```python
from build123d import *
from build123d.topology import SkipClean

# Parameters (mm, degrees)
SKETCH1_R             = 22.146000031
BOSS_EXTRUDE1_DEPTH   = 19.05
SKETCH1_R_2           = 32.595999959
BOSS_EXTRUDE1_2_DEPTH = 19.05
SKETCH1_W             = 304.8
SKETCH1_H             = 304.8
SKETCH1_R_3           = 27.229000025
SKETCH1_R_4           = 38.354
SKETCH1_R_5           = 1.651
BOSS_EXTRUDE1_3_DEPTH = 19.05
SKETCH1_4_R           = 27.229000025
SKETCH1_4_R_2         = 22.146000031
SKETCH1_4_R_3         = 38.354
SKETCH1_4_R_4         = 32.595999959
BOSS_EXTRUDE2_DEPTH   = 12.7
SKETCH1_5_R           = 1.651
CUT_EXTRUDE1_DEPTH    = 12.7
SKETCH5_R             = 2.032
SKETCH5_R_2           = 2.38125
CUT_EXTRUDE2_DEPTH    = 13.7


with BuildPart() as part:
    # Sketch1 → Boss-Extrude1 (new body)
    with BuildSketch(Plane(origin=(0, 0, 0), x_dir=(1, 0, 0), z_dir=(0, 1, 0))):
        with Locations(Location((-11.176, 42.164, 0), (0, 0, 270))):  # turned: the seam where the file's is
            Circle(SKETCH1_R)
    extrude(amount=BOSS_EXTRUDE1_DEPTH)



with BuildPart() as body_2:
    # Sketch1 → Boss-Extrude1 2 (new body)
    with BuildSketch(Plane(origin=(0, 0, 0), x_dir=(1, 0, 0), z_dir=(0, 1, 0))):
        with Locations(Location((61.214, -20.32, 0), (0, 0, 270))):  # turned: the seam where the file's is
            Circle(SKETCH1_R_2)
    extrude(amount=BOSS_EXTRUDE1_2_DEPTH)


with BuildPart() as body_3:
    # Sketch1 → Boss-Extrude1 3 (new body)
    with BuildSketch(Plane(origin=(0, 0, 0), x_dir=(1, 0, 0), z_dir=(0, 1, 0))):
        Rectangle(SKETCH1_W, SKETCH1_H)
        with Locations(Location((-11.176, 42.164, 0), (0, 0, 270))):  # turned: the seam where the file's is
            Circle(SKETCH1_R_3, mode=Mode.SUBTRACT)
        with Locations(Location((61.214, -20.32, 0), (0, 0, 270))):  # turned: the seam where the file's is
            Circle(SKETCH1_R_4, mode=Mode.SUBTRACT)
        with Locations(Location((0, 0, 0), (0, 0, 270))):  # turned: the seam where the file's is
            Circle(SKETCH1_R_5, mode=Mode.SUBTRACT)
    extrude(amount=BOSS_EXTRUDE1_3_DEPTH)


with BuildPart() as part_1:
    with SkipClean():  # keep this step's faces unmerged: merging them makes the solid invalid here
        add(part.part)

        add(body_2.part)  # Boss-Extrude2 merges body 2

        add(body_3.part)  # Boss-Extrude2 merges body 3
        # Sketch1_4 → Boss-Extrude2 (add)
        with BuildSketch(Plane(origin=(0, 0, 0), x_dir=(1, 0, 0), z_dir=(0, 1, 0))):
            with Locations(Location((-11.176, 42.164, 0), (0, 0, 270))):  # turned: the seam where the file's is
                Circle(SKETCH1_4_R)
            with Locations(Location((-11.176, 42.164, 0), (0, 0, 270))):  # turned: the seam where the file's is
                Circle(SKETCH1_4_R_2, mode=Mode.SUBTRACT)
            with Locations(Location((61.214, -20.32, 0), (0, 0, 270))):  # turned: the seam where the file's is
                Circle(SKETCH1_4_R_3)
            with Locations(Location((61.214, -20.32, 0), (0, 0, 270))):  # turned: the seam where the file's is
                Circle(SKETCH1_4_R_4, mode=Mode.SUBTRACT)
            with BuildLine():
                ThreePointArc((99.568, -20.32), (91.665349034, 2.998333088), (71.214, 16.707413034))
                Line((71.214, 16.707413034), (71.214, 10.704171437))
                ThreePointArc((71.214, 10.704171437), (87.562237255, -1.129648079), (93.809999959, -20.32))
                ThreePointArc((93.809999959, -20.32), (42.023648079, -46.668237255), (51.214, 10.704171437))
                Line((51.214, 10.704171437), (51.214, 16.707413034))
                ThreePointArc((51.214, 16.707413034), (37.895666912, -50.771349034), (99.568, -20.32))
            make_face()
            with BuildLine():
                Line((71.214, 10.704171437), (71.214, 16.707413034))
                ThreePointArc((71.214, 16.707413034), (61.214, 18.034), (51.214, 16.707413034))
                Line((51.214, 16.707413034), (51.214, 10.704171437))
                ThreePointArc((51.214, 10.704171437), (61.214, 12.275999959), (71.214, 10.704171437))
            make_face()
            with BuildLine():
                ThreePointArc((-1.176, 67.490240194), (-11.176, 69.393000025), (-21.176, 67.490240194))
                Line((-21.176, 67.490240194), (-21.176, 61.923689202))
                ThreePointArc((-21.176, 61.923689202), (-11.176, 64.310000031), (-1.176, 61.923689202))
                Line((-1.176, 61.923689202), (-1.176, 67.490240194))
            make_face()
            with BuildLine():
                Line((-21.176, 61.923689202), (-21.176, 67.490240194))
                ThreePointArc((-21.176, 67.490240194), (-26.491489579, 19.650576864), (16.053000025, 42.164))
                ThreePointArc((16.053000025, 42.164), (11.337423136, 57.479489579), (-1.176, 67.490240194))
                Line((-1.176, 67.490240194), (-1.176, 61.923689202))
                ThreePointArc((-1.176, 61.923689202), (7.690707684, 53.761096987), (10.970000031, 42.164))
                ThreePointArc((10.970000031, 42.164), (-22.773096987, 23.297292316), (-21.176, 61.923689202))
            make_face()
        extrude(amount=BOSS_EXTRUDE2_DEPTH)

    # Sketch1_5 → Cut-Extrude1 (cut)
    with SkipClean():  # keep this step's faces unmerged: merging them makes the solid invalid here
        with BuildSketch(Plane(origin=(0, 0, 0), x_dir=(1, 0, 0), z_dir=(0, 1, 0))):
            Polygon((-124.40847096, -109.680850921), (-152.4, -109.680850921), (-152.4, -152.4), (-109.680850921, -152.4), (-109.680850921, -124.40847096), align=None)
            with BuildLine():
                ThreePointArc((71.214, 16.707413034), (68.771077011, 30.302427293), (61.747960937, 42.196464709))
                Line((61.747960937, 42.196464709), (25.136544704, 84.689638699))
                ThreePointArc((25.136544704, 84.689638699), (-3.999588367, 92.191814566), (-21.176, 67.490240194))
                Line((-21.176, 67.490240194), (-21.176, 61.923689202))
                ThreePointArc((-21.176, 61.923689202), (-11.176, 64.310000031), (-1.176, 61.923689202))
                Line((-1.176, 61.923689202), (-1.176, 67.490240194))
                ThreePointArc((-1.176, 67.490240194), (2.963287054, 73.442991513), (9.984708116, 71.635066779))
                Line((9.984708116, 71.635066779), (31.14615486, 47.073956315))
                ThreePointArc((31.14615486, 47.073956315), (32.128503793, 44.270491708), (30.940983624, 41.547585342))
                Line((30.940983624, 41.547585342), (-27.66770876, -17.061107042))
                Line((-27.66770876, -17.061107042), (-118.661107042, -17.061107042))
                Line((-118.661107042, -17.061107042), (-118.661107042, -109.680850921))
                Line((-118.661107042, -109.680850921), (-109.680850921, -118.661107042))
                Line((-109.680850921, -118.661107042), (-17.061107042, -118.661107042))
                Line((-17.061107042, -118.661107042), (-17.061107042, -27.66770876))
                Line((-17.061107042, -27.66770876), (40.331599468, 29.72499775))
                ThreePointArc((40.331599468, 29.72499775), (43.35605702, 30.912517919), (46.284134621, 29.504004806))
                Line((46.284134621, 29.504004806), (46.596124349, 29.141892789))
                ThreePointArc((46.596124349, 29.141892789), (50.022253958, 23.339551873), (51.214, 16.707413034))
                Line((51.214, 16.707413034), (51.214, 10.704171437))
                ThreePointArc((51.214, 10.704171437), (61.214, 12.275999959), (71.214, 10.704171437))
                Line((71.214, 10.704171437), (71.214, 16.707413034))
            make_face()
            with Locations(Location((0, 0, 0), (0, 0, 270))):  # turned: the seam where the file's is
                Circle(SKETCH1_5_R, mode=Mode.SUBTRACT)
        extrude(amount=CUT_EXTRUDE1_DEPTH, mode=Mode.SUBTRACT)

    # Sketch5 → Cut-Extrude2 (cut, through all)
    with SkipClean():  # keep this step's faces unmerged: merging them makes the solid invalid here
        with BuildSketch(Plane(origin=(0, 12.7, 0), x_dir=(1, 0, 0), z_dir=(0, 1, 0))):
            with Locations(Location((-11.176, 17.476499972, 0), (0, 0, 270))):  # turned: the seam where the file's is
                Circle(SKETCH5_R)
            with Locations(Location((13.511500028, 42.164, 0), (0, 0, 270))):  # turned: the seam where the file's is
                Circle(SKETCH5_R)
            with Locations(Location((-35.863500028, 42.164, 0), (0, 0, 270))):  # turned: the seam where the file's is
                Circle(SKETCH5_R)
            with Locations(Location((25.739000021, -20.32, 0), (0, 0, 270))):  # turned: the seam where the file's is
                Circle(SKETCH5_R_2)
            with Locations(Location((96.68899998, -20.32, 0), (0, 0, 270))):  # turned: the seam where the file's is
                Circle(SKETCH5_R_2)
            with Locations(Location((61.214, -55.794999979, 0), (0, 0, 270))):  # turned: the seam where the file's is
                Circle(SKETCH5_R_2)
        extrude(amount=-CUT_EXTRUDE2_DEPTH, mode=Mode.SUBTRACT)


solid = part_1.part
```
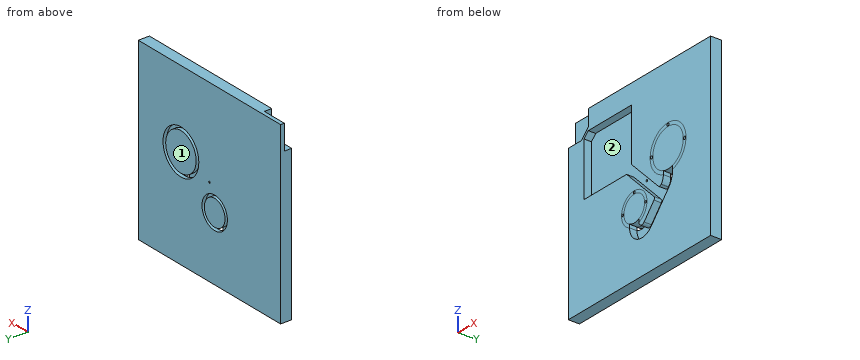
CAD build for the part. Positions are in the model's coordinates, mm. Face numbers are marked on the shaded views. Round coordinates to 2 decimals unless told otherwise and drop trailing zeros. Write each loop counter-clockwise with the first axis right and the second up, starting at its lowest first coordinate (ties: lowest second). Pieces come first, ordered by that corner, then holes.
Item 1: Mould opens along X. For the marked faces 1 and 2 say: released by +X, released by -X, zero draft, split by the parting line, or undercut.
Filled in:
face 1: zero draft
face 2: undercut
Item 2: Band-saw the part on D-D on z = 115. Write the cut outline in (x, y).
Filled in:
outline: (-152.4, 12.7) - (-119.09, 12.7) - (-119.09, 0) - (-113.34, 0) - (-113.34, 12.7) - (-17.06, 12.7) - (-17.06, 0) - (152.4, 0) - (152.4, 19.05) - (-152.4, 19.05) - close
Item 3: Drop flat-ended pins along their axis: pin 1 Ø2.5 at (x, z) = (-35.86, -42.16) entering from +Y; pin 2 Ø6.5 at (y, z) = (5, 143.5) entering from -X; pin 3 Ø5.5 at (x, z) = (25.739, 20.32) entering from -Y. Give the stop position or say it passes through.
Filled in:
pin 1: passes through
pin 2: stops at x = -109.68
pin 3: stops at y = 0
Item 4: Band-saw the part on B-B on x = -103. Write the cut outline in (y, z).
Filled in:
outline: (0, -152.4) - (19.05, -152.4) - (19.05, 152.4) - (0, 152.4) - (0, 118.66) - (12.7, 118.66) - (12.7, 17.06) - (0, 17.06) - close
Item 5: Drill centre lines: L1, parallel to Z at x = -36, y = 5.5; L2, parallel to X at y = 7.25, z = 40; L3, parallel to Z at x = 40, y = 17.25. Where is each one in solid material? Low to high.
Filled in:
L1: z = -152.4 to -44.19, -40.14 to 17.06, 118.66 to 152.4
L2: x = -152.4 to -118.66, -17.06 to 152.4
L3: z = -152.4 to -11.63, -4.43 to 45.07, 52.27 to 152.4
Item 6: Band-saw the part on A-A on z = 83.5. Write the cut outline in (x, y), then the cut area to 3 significant figures.
Filled in:
outline: (-152.4, 0) - (-118.66, 0) - (-118.66, 12.7) - (-17.06, 12.7) - (-17.06, 0) - (152.4, 0) - (152.4, 19.05) - (-152.4, 19.05) - close
area: 4,520 mm2
Item 7: Band-saw the part on C-C on y = 3.5. Give the number of separate pieces and of enclosed holes in the cut face, then the cut area to 3 significant figures.
Filled in:
separate pieces: 1
enclosed holes: 7
area: 77,100 mm2
